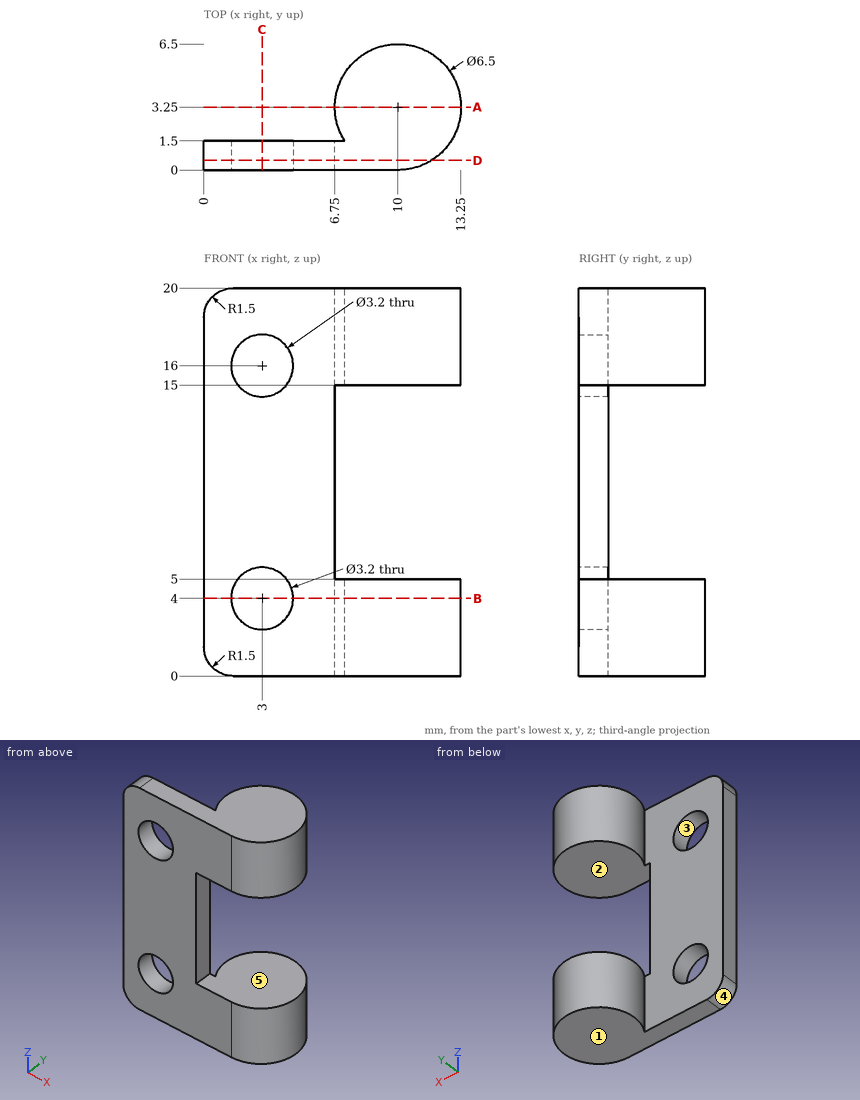
Design review of the part shown in the three views and the two pictorial views. Dimensions are in mm from the part's minimum x, y and z. A direction names the side the tool comes from. Round coordinates to 2 decimals unless told otherwise and drop trailing zeros. Loops run counter-clockwise (first coordinate to the right, second up) from the corner with the lowest first, then second, coordinate; pieces in that order, holes last. Notation, with made-up numbers: (83.5, 2) - (123.5, 2) arc R17 ccw to (123.5, 12) - close; hole circle Ø10 at (-1, 22.25). An arc over 180 degrees is marked (long way). Use one line per item in the form item = value.
1) We need section B-B on z = 4. Write out the cut boundary in (x, y).
Solutions:
outline = (0, 0) - (1.4, 0) - (1.4, 1.5) - (0, 1.5) - close; (4.6, 0) - (10, 0) arc R3.25 ccw (long way) to (7.26, 1.5) - (4.6, 1.5) - close
2) Clearance check with flat-ended pins moving along their axes: P1, Ø1, axis at y = 3.5, z = 11.5, coming from the +X side; P2, Ø5, axis at x = 3, z = 16, coming from the +Y side; P3, Ø1.2, axis at y = 0.5, z = 9, coming from the +X side. State where each tip first meets the part, or that it passes through.
Solutions:
P1 = through
P2 = 1.5
P3 = 6.75
3) We need section A-A on y = 3.25. Write out the cut boundary in (x, z), then the cut area to 3 significant figures.
Solutions:
outline = (6.75, 0) - (13.25, 0) - (13.25, 5) - (6.75, 5) - close; (6.75, 15) - (13.25, 15) - (13.25, 20) - (6.75, 20) - close
area = 65.0 mm2
4) We need section D-D on y = 0.5. Write out the cut boundary in (x, z), then the cut area to 3 significant figures.
Solutions:
outline = (0, 1.5) arc R1.5 ccw to (1.5, 0) - (11.73, 0) - (11.73, 5) - (6.75, 5) - (6.75, 15) - (11.73, 15) - (11.73, 20) - (1.5, 20) arc R1.5 ccw to (0, 18.5) - close; hole circle Ø3.2 at (3, 4); hole circle Ø3.2 at (3, 16)
area = 168 mm2
5) We need section C-C on x = 3. Write out the cut boundary in (y, z).
Solutions:
outline = (0, 0) - (1.5, 0) - (1.5, 2.4) - (0, 2.4) - close; (0, 5.6) - (1.5, 5.6) - (1.5, 14.4) - (0, 14.4) - close; (0, 17.6) - (1.5, 17.6) - (1.5, 20) - (0, 20) - close
6) Wall thickness on probe 1 along Z at (x, y) = (8.75, 4.75); probe 2 along X at (y, z) = (3.25, 16.75); probe 3 along Y at (x, z) = (5, 5.5): over which ranges is each line inside the solid? List them lowest first.
Solutions:
probe_1 = 0 to 5, 15 to 20
probe_2 = 6.75 to 13.25
probe_3 = 0 to 1.5
7) Mouldability with a two-part tool opening along X and no side actions: class the marked faces 3, 4 and 5 as pulls with the +X half, pulls with the -X half, needs draft (parallel to the pull), parting line crosses it, or undercut.
Solutions:
face_3 = undercut
face_4 = pulls with the -X half
face_5 = needs draft
8) Tool access review of the marked faces 1 and 2: name each direction out of +Z, -Z, +X, -X, +Y, -Y from which nothing blocks a thin tool from reaching the whole face with its end or side.
Solutions:
face_1 = -Z, +X, -X, +Y, -Y
face_2 = +X, +Y, -Y
